Autodesk Inventor part; units mm, degrees
ref_plane "YZ Plane" through (0, 0, 0) normal (1, 0, 0) x (0, 1, 0)
ref_plane "XZ Plane" through (0, 0, 0) normal (0, 1, 0) x (-1, 0, 0)
ref_plane "XY Plane" through (0, 0, 0) normal (0, 0, 1) x (1, 0, 0)
sketch "Sketch1" plane through (0, 0, 0) normal (0, 0, 1) x (1, 0, 0)
  arc A0 (2.7781, 11.2277) -> (-2.7781, 11.2277) centre (0, 6.4158) ccw construction
  arc A1 (-2.7781, 11.2277) -> (-5.5562, 6.4158) centre (0, 6.4158) ccw construction
  arc A2 (-5.5562, 6.4158) -> (-2.7781, 1.604) centre (0, 6.4158) ccw construction
  arc A3 (-2.7781, 1.604) -> (2.7781, 1.604) centre (0, 6.4158) ccw construction
  arc A4 (2.7781, 1.604) -> (5.5562, 6.4158) centre (0, 6.4158) ccw construction
  arc A5 (5.5562, 6.4158) -> (2.7781, 11.2277) centre (0, 6.4158) ccw construction
  circle A6 centre (0, 6.4158) radius 3.1376 construction
  arc A7 (65.8645, 106.5408) -> (60.3083, 106.5408) centre (63.0864, 101.729) ccw construction
  arc A8 (60.3083, 106.5408) -> (57.5301, 101.729) centre (63.0864, 101.729) ccw construction
  arc A9 (57.5301, 101.729) -> (60.3083, 96.9171) centre (63.0864, 101.729) ccw construction
  arc A10 (60.3083, 96.9171) -> (65.8645, 96.9171) centre (63.0864, 101.729) ccw construction
  arc A11 (65.8645, 96.9171) -> (68.6426, 101.729) centre (63.0864, 101.729) ccw construction
  arc A12 (68.6426, 101.729) -> (65.8645, 106.5408) centre (63.0864, 101.729) ccw construction
  circle A13 centre (63.0864, 101.729) radius 3.1376 construction
  circle A14 centre (28.0384, 48.7772) radius 16.383 construction
  circle A15 centre (28.0384, 48.7772) radius 18.288
  circle A16 centre (0, 6.4158) radius 6.4158 construction
  circle A17 centre (63.0864, 101.729) radius 6.4158 construction
  circle A18 centre (63.0864, 101.729) radius 6.9238 construction
  circle A19 centre (0, 6.4158) radius 6.9238 construction
  circle A20 centre (0, 6.4158) radius 3.3916
  circle A21 centre (63.0864, 101.729) radius 3.3916
  circle A22 centre (28.0384, 48.7772) radius 38.1 construction
  line L0 (66.9079, 107.5026) -> (-3.8215, 0.6421) construction
  ellipse E0 centre (31.5432, 54.0724) end of major axis (-3.8215, 0.6421) minor radius 35.9584 construction
  circle A23 centre (67.1501, 77.726) radius 3.302
  circle A24 centre (39.4038, 96.091) radius 3.302
  circle A25 centre (19.4364, 4.8439) radius 3.302
  circle A26 centre (-9.0413, 23.6929) radius 3.302
  line L1 (67.1501, 77.726) -> (53.277, 86.9085) construction
  line L2 (39.4038, 96.091) -> (53.277, 86.9085) construction
  line L3 (19.4364, 4.8439) -> (5.1975, 14.2684) construction
  line L4 (-9.0413, 23.6929) -> (5.1975, 14.2684) construction
  circle A27 centre (67.1501, 77.726) radius 10.5597 construction
  circle A28 centre (19.4364, 4.8439) radius 5.715 construction
  circle A29 centre (0, 6.4158) radius 13.7848 construction
  circle A30 centre (63.0864, 101.729) radius 13.7848 construction
  circle A31 centre (19.4364, 4.8439) radius 6.6675 construction
  circle A32 centre (31.5432, 54.0724) radius 64.0738
  point P0 (0, 0)
  point P1 (63.0864, 95.3131)
  point P2 (63.0864, 87.9441)
  point P3 (0, 20.2006)
  dimension "d3" = 0.508
  dimension "d4" = 0.508
  dimension "d0" = 1.905
  dimension "d1" = 0.254
  dimension "d2" = 0.254
  dimension "d6" = 6.604
  dimension "d7" = 6.604
  dimension "d8" = 6.604
  dimension "d9" = 6.604
  dimension "d12" = 11.43
  dimension "d13" = 13.335
extrude "Extrusion1" add sketch "Sketch1" along normal blind 2.2733
equation "\"d2\" = d1"
equation "\"d7\" = d6"
equation "\"d8\" = d6"
equation "\"d9\" = d6"
equation "\"BendRadius\" = Thickness"
equation "\"BendReliefWidth\" = Thickness"
equation "\"BendReliefDepth\" = 0.5 * Thickness"
equation "\"CornerReliefSize\" = 4 * Thickness"
equation "\"MinimumRemnant\" = 2 * Thickness"
equation "\"TransitionRadius\" = BendRadius"
equation "\"JacobiRadiusSize\" = Thickness"
equation "\"GapSize\" = Thickness"
properties part number "Bottom Hub Plate" material "Aluminum"
Build history of the part. All positions in model axes, mm. Coordinates: 2 decimals unless noted, no trailing zeros. Write each loop counter-clockwise with the first axis right and the second up, starting at its lowest first coordinate (ties: lowest second). Pieces come first, ordered by that corner, then holes.
1. Band-saw the part on A-A, the plane x = 0. Give the cut face in (y, z), and give its area (3 significant figures).
Answer block:
outline: (-1.7, 0) - (3.02, 0) - (3.02, 2.27) - (-1.7, 2.27) - close; (9.81, 0) - (109.84, 0) - (109.84, 2.27) - (9.81, 2.27) - close
area: 238 mm2
2. Band-saw the part on C-C, the plane y = 83. Give the cut face in (x, z).
Answer block:
outline: (-25.63, 0) - (88.72, 0) - (88.72, 2.27) - (-25.63, 2.27) - close
3. Drop a flat-ended pin along its axis: pin 1 (1 mm diameter, centred on x = -0.5, z = 0.5, fed in from -Y). Give the stop position or say it passes through.
Answer block:
pin 1: stops at y = -1.7
4. Pull direction Y, two halves, no side cores. Call faces 1 (the cylindrical face through (70.2, 78.99, 1.12)), 2 (the cylindrical face through (-19.304, 93.06, 1.121)), 3 (the flat face through (31, 69, 2.273)): released by +Y, released by -Y, zero draft, split by the parting line, or undercut.
Answer block:
face 1: undercut
face 2: split by the parting line
face 3: zero draft
5. Band-saw the part on B-B, the plane z = 1.35. Give the cut face in (x, y).
Answer block:
outline: circle Ø128.15 at (31.54, 54.07); hole circle Ø6.6 at (-9.04, 23.69); hole circle Ø6.78 at (0, 6.42); hole circle Ø36.58 at (28.04, 48.78); hole circle Ø6.6 at (19.44, 4.84); hole circle Ø6.6 at (39.4, 96.09); hole circle Ø6.78 at (63.09, 101.73); hole circle Ø6.6 at (67.15, 77.73)
6. Band-saw the part on D-D, the plane x = 81.5. Give the cut face in (y, z), and give its area (3 significant figures).
Answer block:
outline: (13.95, 0) - (94.19, 0) - (94.19, 2.27) - (13.95, 2.27) - close
area: 182 mm2
7. Drill centre lines: probe 1 along X at (y, z) = (7.5, 0.3); probe 2 along Y at (x, z) = (25.5, 0.8); probe 3 along Y at (x, z) = (65.5, 1). Where is each one in solid material? Low to high.
Answer block:
probe 1: x = -12.46 to -3.21, 3.21 to 17.47, 21.4 to 75.55
probe 2: y = -9.72 to 30.67, 66.89 to 117.86
probe 3: y = -0.26 to 74.87, 80.59 to 99.35, 104.11 to 108.41
